Source: three-view drawing plus pictorial views. Frame: mm from the lowest corner of the part. A direction names the side the tool comes from. Coordinates: 2 decimals unless noted, no trailing zeros. Order: outer loops, then holes, each group sorted by start corner. A loop starts at its lowest first (then second) coordinate and runs counter-clockwise, first axis right, second up. Notation, with made-up numbers: (-0.5, 52.5) -> (51.5, 52.5) arc R28 ccw to (51.5, 74.5) -> close; hole circle Ø2 at (66, -27.75). An arc over 180 degrees is marked (long way). Use one line per item in the form item = value. Start each with the question number.
1) Ray query, line 1 along Y through (x, z) = (11, 0.1); line 2 along Z through (x, y) = (16.5, 10); line 3 along Y through (x, z) = (10.25, 0.65). Return the intervals inside material, ascending.
2) Section query C-C on z = 1.1. Output: boundary loops of the cut face in (x, y).
3) Section query A-A on y = 11. Output: boundary loops of the cut face in (x, z).
4) Pin query (flat end, axial travel): pin 1 (8 mm diameter, centred on x = 11, y = 7.5, fed in from -Z); pin 2 (1.5 mm diameter, centred on x = 8.5, z = 1, fed in from +Y). Return the tip coordinate at first contact, or that it passes through.
5) Access query for the marked faces 1 and 2. Directions: +Z, -Z, +X, -X, +Y, -Y. A direction counts if a zero-diameter tool reaches every point of the face in a straight line with its end or side. Return the directions, or none.
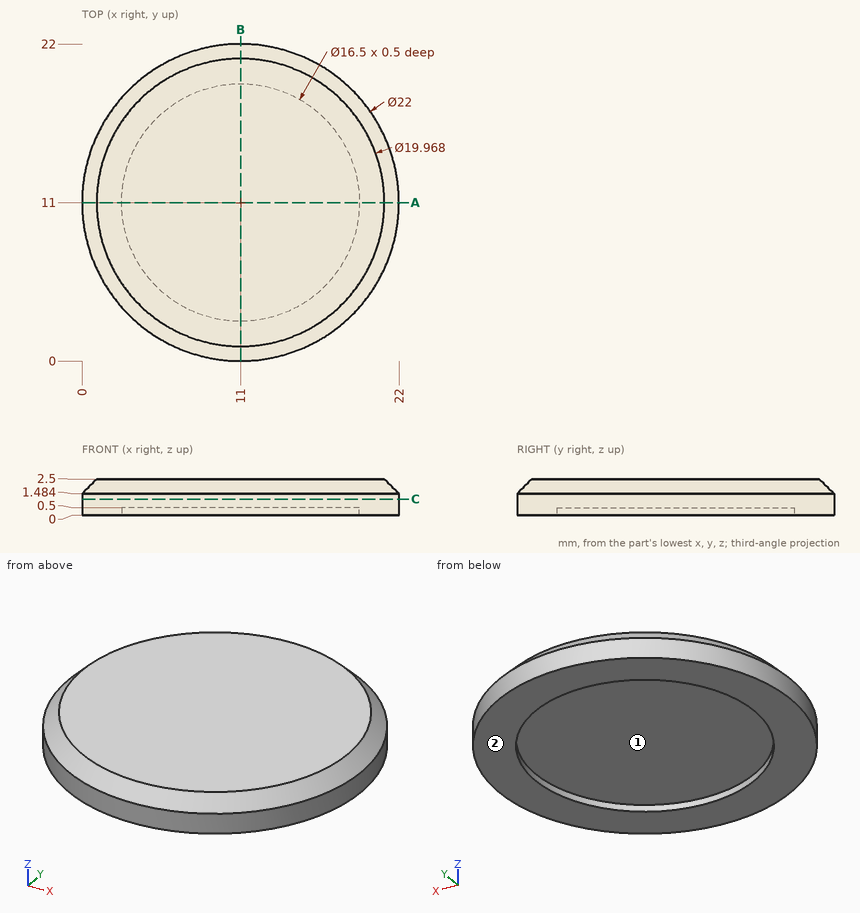
Answers below:
q1.line_1 = 0 to 2.75, 19.25 to 22
q1.line_2 = 0.5 to 2.5
q1.line_3 = 0.03 to 21.97
q2.outline = circle Ø22 at (11, 11)
q3.outline = (0, 0) -> (2.75, 0) -> (2.75, 0.5) -> (19.25, 0.5) -> (19.25, 0) -> (22, 0) -> (22, 1.48) -> (20.98, 2.5) -> (1.02, 2.5) -> (0, 1.48) -> close
q4.pin_1 = 0.5
q4.pin_2 = 21.86
q5.face_1 = -Z
q5.face_2 = -Z, +X, -X, +Y, -Y
